Here's how the part is built. I have some questions about the finished solid (model axes, mm). A direction names the side the tool comes from. Round coordinates to 2 decimals unless told otherwise and drop trailing zeros. Order: outer loops, then holes, each group sorted by start corner. A loop starts at its lowest first (then second) coordinate and runs counter-clockwise, first axis right, second up. Notation, with made-up numbers: (15.25, 29) -> (55.25, 29) arc R28 ccw to (55.25, 58) -> close; hole circle Ø7 at (59.5, 29). An arc over 180 degrees is marked (long way). Answer in a Markdown table with one row per item.
```python
from build123d import *

# Parameters (mm, degrees)
CONTACT_DEPTH = 0.3
CHAMFER1_SIZE = 0.1
PLASTIC_DEPTH = 2.54


with BuildPart() as part:
    # Sketch2 → Contact (new, symmetric)
    with BuildSketch(Plane(origin=(0, 0, 0), x_dir=(0, -1, 0), z_dir=(1, 0, 0))):
        with BuildLine():
            Line((0.3, 3.2), (-0.3, 3.2))
            Line((-0.3, 3.2), (-0.3, -0.67))
            ThreePointArc((-0.3, -0.67), (-0.387867966, -0.882132034), (-0.6, -0.97))
            Line((-0.6, -0.97), (-10.5, -0.97))
            Line((-10.5, -0.97), (-10.5, -1.57))
            Line((-10.5, -1.57), (-0.6, -1.57))
            ThreePointArc((-0.6, -1.57), (0.036396103, -1.306396103), (0.3, -0.67))
            Line((0.3, -0.67), (0.3, 3.2))
        make_face()
    extrude(amount=CONTACT_DEPTH, both=True)

    # Chamfer1
    chamfer1_edges = [part.edges().sort_by_distance(p)[0] for p in [
        (0.3, 10.5, 1.27),
        (0, 0.3, -3.2),
        (0, -0.3, -3.2),
        (0, 10.5, 1.57),
        (0, 10.5, 0.97),
        (0.3, 0, -3.2),
        (-0.3, 0, -3.2),
        (-0.3, 10.5, 1.27),
    ]]
    chamfer(chamfer1_edges, length=CHAMFER1_SIZE)

    # Sketch1 → Plastic (add)
    with BuildSketch(Plane(origin=(0, 4.3, 0), x_dir=(0, 0, -1), z_dir=(0, 1, 0))):
        Polygon((-2.04, 1.27), (-0.5, 1.27), (0, 0.77), (0, -0.77), (-0.5, -1.27), (-2.04, -1.27), (-2.54, -0.77), (-2.54, 0.77), align=None)
    extrude(amount=-PLASTIC_DEPTH)


solid = part.part
```
1. Suppose I cut it at B-B on x = 0.1. Write out the boundary of the cut face in (y, z).
Numbers:
| item | result |
|---|---|
| outline | (-0.3, -3.1) -> (-0.2, -3.2) -> (0.2, -3.2) -> (0.3, -3.1) -> (0.3, 0.67) arc R0.3 cw to (0.6, 0.97) -> (1.76, 0.97) -> (1.76, 0) -> (4.3, 0) -> (4.3, 0.97) -> (10.4, 0.97) -> (10.5, 1.07) -> (10.5, 1.47) -> (10.4, 1.57) -> (4.3, 1.57) -> (4.3, 2.54) -> (1.76, 2.54) -> (1.76, 1.57) -> (0.6, 1.57) arc R0.9 ccw to (-0.3, 0.67) -> close |
2. For pin 1 Ø0.8 at (x, z) = (0.5, 1.5) entering from +Y; pin 2 Ø1 at (x, y) = (-1, 6.5) entering from -Z; pin 3 Ø0.8 at (x, z) = (0.5, 1.5) entering from -Y; pin 4 Ø0.5 at (y, z) = (8.5, 1) entering from -X, each with a flat end and sliding along its axis, tell me the tip position at first contact or that it passes through.
Numbers:
| item | result |
|---|---|
| pin 1 | stops at y = 10.5 |
| pin 2 | passes through |
| pin 3 | stops at y = -0.16 |
| pin 4 | stops at x = -0.3 |
3. Suppose I cut it at A-A on z = 0.1. Write out the boundary of the cut face in (x, y), then the cut area to 3 significant figures.
Numbers:
| item | result |
|---|---|
| outline | (-0.87, 1.76) -> (0.87, 1.76) -> (0.87, 4.3) -> (-0.87, 4.3) -> close; (-0.3, -0.3) -> (0.3, -0.3) -> (0.3, 0.3) -> (-0.3, 0.3) -> close |
| area | 4.78 mm2 |
4. For faces 1 (the face through (-0.3, 0, 0)), 2 (the face through (1.27, 3, 1)), 3 (the face through (0, 3, 0)), 4 (the face through (0.3, 0, 0)), which set-ups out of +Z, -Z, +X, -X, +Y, -Y let a thin tool reach every point of the face, with its end or its side?
Numbers:
| item | result |
|---|---|
| face 1 | +Z, -Z, -X, -Y |
| face 2 | +Z, -Z, +X, +Y, -Y |
| face 3 | -Z, +X, -X, +Y |
| face 4 | +Z, -Z, +X, -Y |
5. Please list where these lines run through material, in increasing order: line 1 along Z through (x, y) = (-0.1, 7); line 2 along Y through (x, z) = (-0.45, 0.85); line 3 along Z through (x, y) = (-0.15, 3.75).
Numbers:
| item | result |
|---|---|
| line 1 | z = 0.97 to 1.57 |
| line 2 | y = 1.76 to 4.3 |
| line 3 | z = 0 to 2.54 |
6. Suppose I cut it at D-D on z = -1.2. Write out the boundary of the cut face in (x, y).
Numbers:
| item | result |
|---|---|
| outline | (-0.3, -0.3) -> (0.3, -0.3) -> (0.3, 0.3) -> (-0.3, 0.3) -> close |
7. Suppose I cut it at C-C on y = 3.25. Write out the boundary of the cut face in (x, z).
Numbers:
| item | result |
|---|---|
| outline | (-1.27, 0.5) -> (-0.77, 0) -> (0.77, 0) -> (1.27, 0.5) -> (1.27, 2.04) -> (0.77, 2.54) -> (-0.77, 2.54) -> (-1.27, 2.04) -> close |
